Could you check a few things on this model? Use its own coordinates, in mm. A direction names the side the tool comes from. Coordinates: 2 decimals unless noted, no trailing zeros. Loops run counter-clockwise (first coordinate to the right, second up) from the corner with the lowest first, then second, coordinate; pieces in that order, holes last.
1) If I drill on line 1 along Y through (x, z) = (124.5, -5.75); line 2 along X through (y, z) = (96, -5); line 3 along Z through (x, y) = (129, 81.5), over which ranges is the centre line in solid material (lowest first)?
2) Imagine slicing it at A-A on z = -9. Please give me the cut outline in (x, y).
3) Thinking about a two-plate mould opening in X: for faces 1 (the face through (125, 106.96, -11)), 2 (the face through (125, 83.131, -5)), 3 (the face through (114.736, 92, -11)), which applies, released by +X, released by -X, zero draft, split by the parting line, or undercut?
4) Imagine slicing it at D-D on y = 92.25. Please give me the cut outline in (x, z), plus the area to 3 significant figures.
5) Imagine slicing it at B-B on x = 122.5. Please give me the cut outline in (y, z).
6) Will this pin go through, and if not, where does the flat tip stop? P1, Ø2.5, axis at x = 126.5, y = 101.5, coming from the +Z side.
7) Imagine slicing it at C-C on y = 82.5. Please give me the cut outline in (x, z).
8) For faces 4 (the face through (117.263, 82, -5)), 5 (the face through (125, 76.96, -11)), which set-ups out of +Z, -Z, +X, -X, +Y, -Y let a thin tool reach every point of the face, with its end or its side?
```python
from build123d import *

# Parameters (mm, degrees)
SKETCH_1_W      = 20.3
SKETCH_1_H      = 30
SKETCH_1_W_2    = 12.8
SKETCH_1_H_2    = 5.2
EXTRUDE_1_DEPTH = 10
SKETCH_2_W      = 20.3
SKETCH_2_H      = 30
EXTRUDE_2_DEPTH = 12


with BuildPart() as part:
    # Эскиз1 → Бобышка-Вытянуть1 (new body)
    with BuildSketch(Plane.XY):
        with Locations((124.886360731, 91.960324966)):
            Rectangle(SKETCH_1_W, SKETCH_1_H)
        with Locations((124.886360731, 93.560324966)):
            Rectangle(SKETCH_1_W_2, SKETCH_1_H_2, mode=Mode.SUBTRACT)
        with Locations((124.886360731, 102.660324966)):
            Rectangle(SKETCH_1_W_2, SKETCH_1_H_2, mode=Mode.SUBTRACT)
        Polygon((129.566618584, 77.960324966), (120.129531537, 77.960324966), (117.26298197, 80.238017172), (117.26298197, 83.13068263), (132.886839219, 83.13068263), (132.886839219, 79.296578456), align=None, mode=Mode.SUBTRACT)
    extrude(amount=-EXTRUDE_1_DEPTH)

    # Эскиз2 → Бобышка-Вытянуть2 (add)
    with BuildSketch(Plane(origin=(0, 0, -10), x_dir=(-1, 0, 0), z_dir=(0, 0, -1))):
        with Locations((-124.886360731, 91.960324966)):
            Rectangle(SKETCH_2_W, SKETCH_2_H)
    extrude(amount=EXTRUDE_2_DEPTH)


solid = part.part
```
Filled in:
1. line 1: y = 76.96 to 77.96, 83.13 to 90.96, 96.16 to 100.06, 105.26 to 106.96
1. line 2: x = 114.74 to 118.49, 131.29 to 135.04
1. line 3: z = -22 to -10
2. outline: (114.74, 76.96) - (135.04, 76.96) - (135.04, 106.96) - (114.74, 106.96) - close; hole (117.26, 80.24) - (120.13, 77.96) - (129.57, 77.96) - (132.89, 79.3) - (132.89, 83.13) - (117.26, 83.13) - close; hole (118.49, 90.96) - (131.29, 90.96) - (131.29, 96.16) - (118.49, 96.16) - close; hole (118.49, 100.06) - (131.29, 100.06) - (131.29, 105.26) - (118.49, 105.26) - close
3. face 1: zero draft
3. face 2: undercut
3. face 3: released by -X
4. outline: (114.74, -22) - (135.04, -22) - (135.04, 0) - (131.29, 0) - (131.29, -10) - (118.49, -10) - (118.49, 0) - (114.74, 0) - close
4. area: 319 mm2
5. outline: (76.96, -22) - (106.96, -22) - (106.96, 0) - (105.26, 0) - (105.26, -10) - (100.06, -10) - (100.06, 0) - (96.16, 0) - (96.16, -10) - (90.96, -10) - (90.96, 0) - (83.13, 0) - (83.13, -10) - (77.96, -10) - (77.96, 0) - (76.96, 0) - close
6. P1: stops at z = -10
7. outline: (114.74, -22) - (135.04, -22) - (135.04, 0) - (132.89, 0) - (132.89, -10) - (117.26, -10) - (117.26, 0) - (114.74, 0) - close
8. face 4: +Z
8. face 5: +Z, -Z, +X, -X, -Y
